Can you work these out from the model? Positions are in its coordinate system, mm. Face numbers are marked on the shaded views. Give positions to 0.01 mm unless a question says otherwise; leave off trailing zeros. Loops run counter-clockwise (first coordinate to the right, second up) from the corner with the lowest first, then second, coordinate; pieces in that order, holes last. Notation, with made-up numbers: M 29,-32 L 66,-32 A25 ccw 66,-13 Z; hole C -3.5,16 d6. An arc over 180 degrees is marked long. Use CSV: the item, a comma, the result in double quotes.
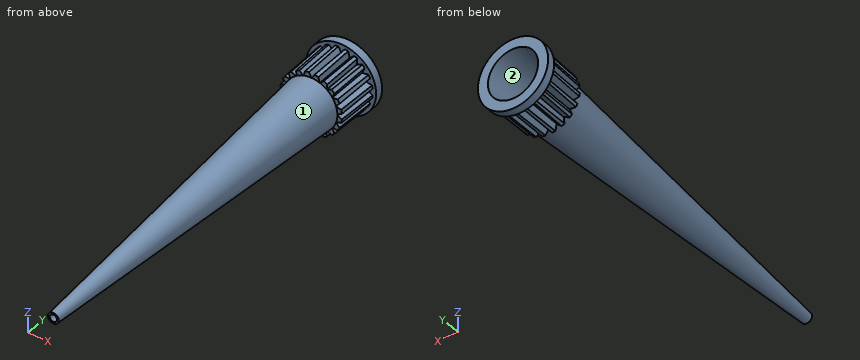
from build123d import *

# Parameters (mm, degrees)
IZIM2_R               = 3
KES_EKSTR_ZYON1_DEPTH = 49
KES_EKSTR_ZYON1_DRAFT = -3
KES_EKSTR_ZYON4_DEPTH = 5


with BuildPart() as part:
    # Çizim1 → Döndür1 (revolve)
    with BuildSketch(Plane.XY, mode=Mode.PRIVATE) as d_nd_r1_sk:
        Polygon((0, 0), (0, 49), (4.2, 49), (4.2, 48), (3.8, 48), (3.7, 43), (3.15, 43), (0.65, 0), align=None)
    revolve(d_nd_r1_sk.sketch.rotate(Axis((0, 0, 0), (0, 1, 0)), 90), axis=Axis((0, 0, 0), (0, 1, 0)))


with BuildPart() as kes_ekstr_zyon1_tool:
    # Çizim2 → Kes-Ekstrüzyon1 (with draft: the straight prism first)
    with BuildSketch(Plane(origin=(0, 49, 0), x_dir=(1, 0, 0), z_dir=(0, 1, 0))):
        Circle(IZIM2_R)
    extrude(amount=-KES_EKSTR_ZYON1_DEPTH)
    # Kes-Ekstrüzyon1: the draft: its side faces are tilted about the plane it starts from
    kes_ekstr_zyon1_sides = [kes_ekstr_zyon1_tool.faces().sort_by_distance(p)[0] for p in [
        (-3, 24.5, 0),
    ]]
    draft(kes_ekstr_zyon1_sides, Plane(origin=(0, 49, 0), x_dir=(1, 0, 0), z_dir=(0, 1, 0)), KES_EKSTR_ZYON1_DRAFT)


with BuildPart() as part_1:
    add(part.part)

    # Kes-Ekstrüzyon1: cut by kes_ekstr_zyon1_tool
    add(kes_ekstr_zyon1_tool.part, mode=Mode.SUBTRACT)

    # Çizim3 → Kes-Ekstrüzyon4 (cut)
    with BuildSketch(Plane.XZ.offset(-43)):
        Polygon((0.08224501, 3.1), (-0.41775499, 3.966025404), (0.58224501, 3.966025404), align=None)
        Polygon((0.815256969, 3.918905719), (1.766313485, 3.609888725), (1.02316866, 2.940758119), align=None)
        Polygon((1.973360244, 3.493070587), (2.782377238, 2.905285335), (1.868831781, 2.498548692), align=None)
        Polygon((2.943191617, 2.730203716), (3.53097687, 1.921186722), (2.536454974, 1.816658258), align=None)
        Polygon((3.629817237, 1.704979831), (3.938834232, 0.753923315), (2.960686631, 0.961835006), align=None)
        Polygon((3.966025404, 0.51775499), (3.966025404, -0.48224501), (3.1, 0.01775499), align=None)
        Polygon((3.918905719, -0.715256969), (3.609888725, -1.666313485), (2.940758119, -0.92316866), align=None)
        Polygon((3.493070587, -1.873360244), (2.905285335, -2.682377238), (2.498548692, -1.768831781), align=None)
        Polygon((2.730203716, -2.843191617), (1.921186722, -3.43097687), (1.816658258, -2.436454974), align=None)
        Polygon((1.704979831, -3.529817237), (0.753923315, -3.838834232), (0.961835006, -2.860686631), align=None)
        Polygon((0.51775499, -3.866025404), (-0.48224501, -3.866025404), (0.01775499, -3), align=None)
        Polygon((-0.715256969, -3.818905719), (-1.666313485, -3.509888725), (-0.92316866, -2.840758119), align=None)
        Polygon((-1.873360244, -3.393070587), (-2.682377238, -2.805285335), (-1.768831781, -2.398548692), align=None)
        Polygon((-2.843191617, -2.630203716), (-3.43097687, -1.821186722), (-2.436454974, -1.716658258), align=None)
        Polygon((-3.529817237, -1.604979831), (-3.838834232, -0.653923315), (-2.860686631, -0.861835006), align=None)
        Polygon((-3.866025404, -0.41775499), (-3.866025404, 0.58224501), (-3, 0.08224501), align=None)
        Polygon((-3.818905719, 0.815256969), (-3.509888725, 1.766313485), (-2.840758119, 1.02316866), align=None)
        Polygon((-3.393070587, 1.973360244), (-2.805285335, 2.782377238), (-2.398548692, 1.868831781), align=None)
        Polygon((-2.630203716, 2.943191617), (-1.821186722, 3.53097687), (-1.716658258, 2.536454974), align=None)
        Polygon((-1.604979831, 3.629817237), (-0.653923315, 3.938834232), (-0.861835006, 2.960686631), align=None)
    extrude(amount=-KES_EKSTR_ZYON4_DEPTH, mode=Mode.SUBTRACT)


solid = part_1.part
Q1. Please list where these lines run through material, in increasing order: L1, parallel to X at y = 33, z = -1; L2, parallel to Z at x = -0.5, y = 40; L3, parallel to Z at x = 1.5, y = 45.5. Write a range as from..to.
Model answer:
L1,"-2.37..-1.92, 1.92..2.37"
L2,"-2.93..-2.48, 2.48..2.93"
L3,"-3.35..-2.38, 2.38..3.37"
Q2. I want a section at B-B, the plane y = 6. Please give me the cut outline in (x, z).
Model answer:
outline,"C 0,0 d2; hole C 0,0 d1.49"
Q3. If we mould it in two halves opening along X, with no side actions, what happens to the marked faces 1 and 2? For each: released by +X, released by -X, zero draft, split by the parting line, or undercut.
Model answer:
face 1,"split by the parting line"
face 2,"undercut"
Q4. I'm going to push flat-ended pins straight in: P1, Ø4, axis at x = 2.5, y = 5, coming from the -Z side; P2, Ø0.7, axis at x = -3.5, z = 1, coming from the -Y side; P3, Ø5, axis at y = 36, z = -1, coming from the -X side. Where does each tip first touch, or does it pass through?
Model answer:
P1,"z = -0.8"
P2,"y = 43"
P3,"x = -2.88"
Q5. I want a section at A-A, the plane y = 20.5. Please give me the cut outline in (x, z).
Model answer:
outline,"C 0,0 d3.68; hole C 0,0 d3.01"
